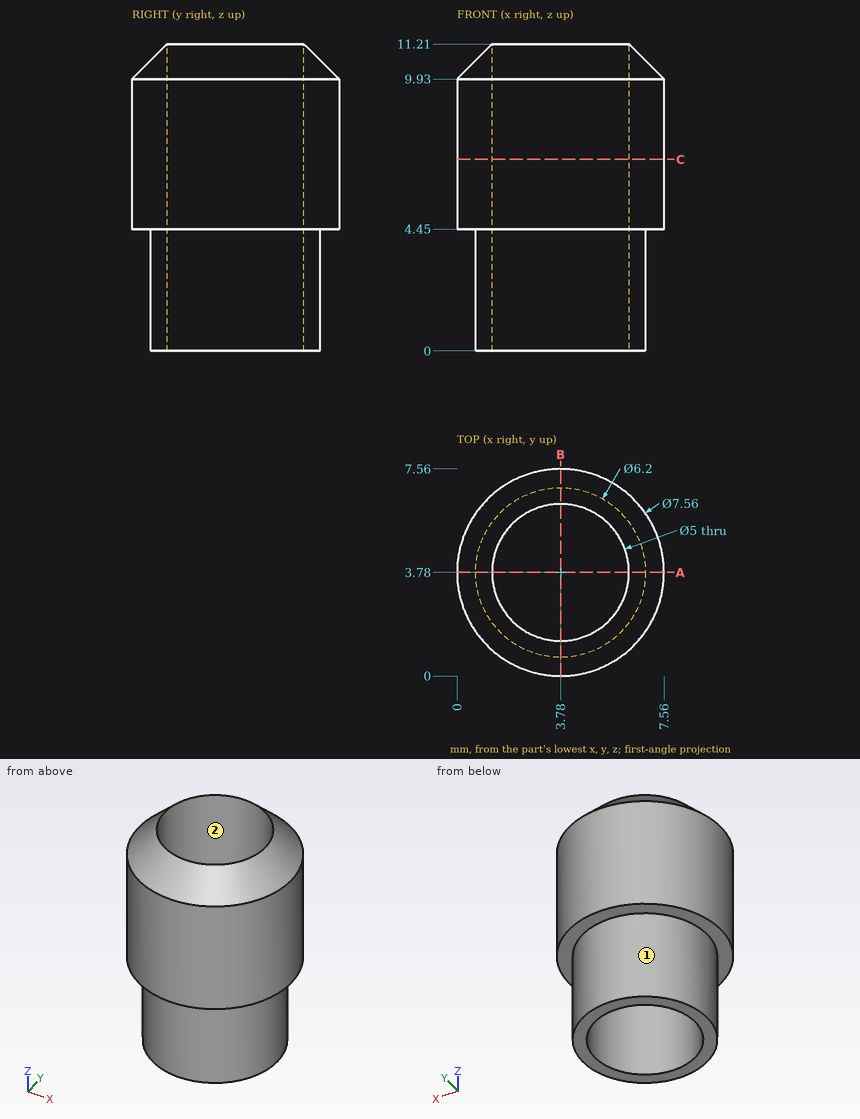
Could you check a few things on this drawing? It's one solid part, dimensions in mm from its lowest x, y, z. Coordinates: 2 decimals unless noted, no trailing zeros. Order: outer loops, then holes, each group sorted by start corner. A loop starts at its lowest first (then second) coordinate and runs counter-clockwise, first axis right, second up. Notation, with made-up numbers: (82, -27) - (120, -27) arc R37 ccw to (120, 12) - close; hole circle Ø6 at (45.5, 0). An arc over 180 degrees is marked (long way). Answer as a JSON object with one key per item and string values. Group by question number.
Q1. Will these pins go through, and if not, where does the flat tip stop? P1, Ø1.5, axis at x = 5.5, z = 9.5, coming from the -Y side; P2, Ø4, axis at y = 1.5, z = 1.5, coming from the -X side; P3, Ø4, axis at x = 6, z = 1.5, coming from the -Y side.
Q2. Imagine slicing it at C-C (z = 7). Please give me the cut outline in (x, y).
Q3. I need wall thicknesses on line 1 (Y direction, x = 3.78, z = 6.5); line 2 (Y direction, x = 3.78, z = 4); line 3 (X direction, y = 2, z = 1.75). Which ranges of each line are inside material? Lowest first, please. Write a range as from..to.
Q4. We'd pull the mould along Y, two halves only. Please class the marked faces 1 and 2: +Y half, -Y half, draft (parallel to the pull), parting line (faces both ways), or undercut.
Q5. Imagine slicing it at A-A (y = 3.78). Please give me the cut outline in (x, z), and give its area (3 significant figures).
Determined:
{
 "1": {"P1": "stops at y = 0.13", "P2": "stops at x = 0.69", "P3": "stops at y = 0.69"},
 "2": {"outline": "circle Ø7.56 at (3.78, 3.78); hole circle Ø5 at (3.78, 3.78)"},
 "3": {"line 1": "y = 0..1.28, 6.28..7.56", "line 2": "y = 0.68..1.28, 6.28..6.88", "line 3": "x = 1.24..2.02, 5.54..6.32"},
 "4": {"face 1": "parting line", "face 2": "undercut"},
 "5": {"outline": "(0, 4.45) - (0.68, 4.45) - (0.68, 0) - (1.28, 0) - (1.28, 11.21) - (0, 9.93) - close; (6.28, 0) - (6.88, 0) - (6.88, 4.45) - (7.56, 4.45) - (7.56, 9.93) - (6.28, 11.21) - close", "area": "21.0 mm2"}
}
